from build123d import *

# Parameters (mm, degrees)
SKETCH1_R           = 2.2
BOSS_EXTRUDE1_DEPTH = 12
SKETCH3_R           = 4
BOSS_EXTRUDE2_DEPTH = 7


with BuildPart() as part:
    # Sketch1 → Boss-Extrude1 (new body)
    with BuildSketch(Plane(origin=(0, 0, 0), x_dir=(1, 0, 0), z_dir=(0, 1, 0))):
        Circle(SKETCH1_R)
    extrude(amount=BOSS_EXTRUDE1_DEPTH)

    # Sketch3 → Boss-Extrude2 (add)
    with BuildSketch(Plane(origin=(0, 12, 0), x_dir=(1, 0, 0), z_dir=(0, 1, 0))):
        Circle(SKETCH3_R)
    extrude(amount=BOSS_EXTRUDE2_DEPTH)

    # Sketch4 → Revolve2 (revolve)
    with BuildSketch(Plane.XY):
        with BuildLine():
            Line((0, 28.11938617), (0, 19))
            Line((0, 19), (4, 19))
            ThreePointArc((4, 19), (5.676610407, 25.69672264), (0, 29.62523519))
            Line((0, 29.62523519), (0, 28.11938617))
        make_face()
    revolve(axis=Axis((0, 28.11938617, 0), (0, -1, 0)))


solid = part.part
Here's how the part is built. I have some questions about the finished solid (model axes, mm). A direction names the side the tool comes from. Coordinates: 2 decimals unless noted, no trailing zeros. Write each loop counter-clockwise with the first axis right and the second up, starting at its lowest first coordinate (ties: lowest second). Pieces come first, ordered by that corner, then holes. Notation, with made-up numbers: (-3, 26) - (45, 26) arc R24 cw to (45, 55) - close; hole circle Ø7 at (15, 69). An arc over 180 degrees is marked (long way). Use one line per item in the form item = value.
1) Suppose I cut it at D-D, the plane x = 1.5. Write out the boundary of the cut face in (y, z), plus the area to 3 significant figures.
Solved:
outline = (0, -1.61) - (12, -1.61) - (12, -3.71) - (19, -3.71) arc R5.88 ccw (long way) to (19, 3.71) - (12, 3.71) - (12, 1.61) - (0, 1.61) - close
area = 192 mm2
2) Suppose I cut it at A-A, the plane x = 0. Write out the boundary of the cut face in (y, z).
Solved:
outline = (0, -2.2) - (12, -2.2) - (12, -4) - (19, -4) arc R6.07 ccw (long way) to (19, 4) - (12, 4) - (12, 2.2) - (0, 2.2) - close
3) I need wall thicknesses on line 1 (X direction, y = 9.25, z = 0); line 2 (X direction, y = 8.75, z = 2); line 3 (Y direction, x = -3.5, z = -1.25). Which ranges of each line are inside material? Lowest first, please.
Solved:
line_1 = -2.2 to 2.2
line_2 = -0.92 to 0.92
line_3 = 12 to 28.35
4) I'm going to push flat-ended pins straight in: P1, Ø2, axis at y = 6, z = 2.5, coming from the +X side; P2, Ø1, axis at x = 2, z = 2.5, coming from the -Y side; P3, Ø4, axis at x = -2, y = 13, coming from the -Z side; P4, Ø1, axis at x = 3.5, y = 8.5, coming from the +Z side. Where does each tip first touch, or does it pass through?
Solved:
P1 = 1.61
P2 = 12
P3 = -4
P4 = through
5) Suppose I cut it at B-B, the plane z = 0. Write out the boundary of the cut face in (x, y).
Solved:
outline = (-4, 12) - (-2.2, 12) - (-2.2, 0) - (2.2, 0) - (2.2, 12) - (4, 12) - (4, 19) arc R6.07 ccw (long way) to (-4, 19) - close
6) On a 3-axis mill with a long thin cutter (end or side, diameter ignored), from which of +Z, -Z, +X, -X, +Y, -Y can I reach the whole of each face in a straight line? I mean faces 1 (the flat face through (0, 0, 0)), 2 (the cylindrical face through (2.1, 5.92, -0.66)). Say none if no direction works.
Solved:
face_1 = +Z, -Z, +X, -X, -Y
face_2 = -Y
7) Suppose I cut it at C-C, the plane y = 12.5. Write out the boundary of the cut face in (x, z), plus the area to 3 significant figures.
Solved:
outline = circle Ø8 at (0, 0)
area = 50.3 mm2
